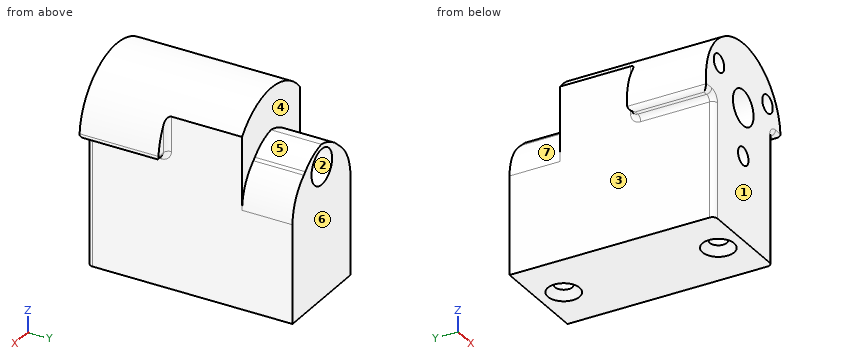
```python
from build123d import *

# Parameters (mm, degrees)
SKETCH2_R                                      = 12.7
BOSS_EXTRUDE6_DEPTH                            = 40.64
SKETCH3_R                                      = 3.5
CUT_EXTRUDE1_DEPTH                             = 40.64
SKETCH4_R                                      = 1.778
CUT_EXTRUDE2_DEPTH                             = 6
BOSS_EXTRUDE8_DEPTH                            = 10
SKETCH8_W                                      = 25.185693912
SKETCH8_H                                      = 10
BOSS_EXTRUDE9_DEPTH                            = 7.284789049
BOSS_EXTRUDE10_DEPTH                           = 30.64
CSK_FOR_M3_FLAT_HEAD_MACHINE_SCREW1_AT_2_COUNT = 2
CSK_FOR_M3_FLAT_HEAD_MACHINE_SCREW1_AT_2_PITCH = 9.039543014
CSK_FOR_M3_FLAT_HEAD_MACHINE_SCREW1_AT_3_COUNT = 2
CSK_FOR_M3_FLAT_HEAD_MACHINE_SCREW1_AT_3_PITCH = 9.039543014
SKETCH16_W                                     = 3.769994858
SKETCH16_H                                     = 22.000968128
CUT_EXTRUDE3_DEPTH                             = 25
SKETCH17_W                                     = 10.276759259
SKETCH17_H                                     = 15.64
CUT_EXTRUDE4_DEPTH                             = 2.743753899
SKETCH18_W                                     = 12.6
SKETCH18_H                                     = 15.64
CUT_EXTRUDE5_DEPTH                             = 2.743753899
SKETCH20_W                                     = 2.743753899
SKETCH20_H                                     = 13.478747573
CUT_EXTRUDE7_DEPTH                             = 25
SKETCH21_W                                     = 5.741451758
SKETCH21_H                                     = 11.696500392
SKETCH21_W_2                                   = 5.938790765
BOSS_EXTRUDE12_DEPTH                           = 15
CUT_EXTRUDE8_START                             = -10
CUT_EXTRUDE8_DEPTH                             = 10
FILLET1_R                                      = 10
FILLET5_R                                      = 10
SKETCH23_W                                     = 2.743753899
SKETCH23_H                                     = 13.478747573
CUT_EXTRUDE9_DEPTH                             = 20
SKETCH24_W                                     = 5.557541457
SKETCH24_H                                     = 9.320824694
SKETCH24_W_2                                   = 5.259690838
BOSS_EXTRUDE13_DEPTH                           = 20
FILLET6_R                                      = 1


with BuildPart() as part:
    # Sketch2 → Boss-Extrude6 (new body)
    with BuildSketch(Plane(origin=(0, -2111.389926236, 0), x_dir=(1, 0, 0), z_dir=(0, 1, 0))):
        with Locations(Location((-53.693967541, 163.840329354, 0), (0, 0, 180))):
            Circle(SKETCH2_R)
    extrude(amount=BOSS_EXTRUDE6_DEPTH)

    # Sketch3 → Cut-Extrude1 (cut)
    with BuildSketch(Plane(origin=(0, -2070.749926236, 0), x_dir=(1, 0, 0), z_dir=(0, 1, 0))):
        with Locations(Location((-53.693967541, 163.840329354, 0), (0, 0, 270))):
            Circle(SKETCH3_R)
    extrude(amount=-CUT_EXTRUDE1_DEPTH, mode=Mode.SUBTRACT)

    # Sketch4 → Cut-Extrude2 (cut)
    with BuildSketch(Plane.XZ.offset(2111.389926236)):
        with Locations(Location((-61.942859512, -159.077829354, 0), (0, 0, 270))):
            Circle(SKETCH4_R)
        with Locations(Location((-53.693967541, -173.365329354, 0), (0, 0, 270))):
            Circle(SKETCH4_R)
        with Locations(Location((-45.44507557, -159.077829354, 0), (0, 0, 270))):
            Circle(SKETCH4_R)
    extrude(amount=-CUT_EXTRUDE2_DEPTH, mode=Mode.SUBTRACT)

    # Sketch7 → Boss-Extrude8 (add)
    with BuildSketch(Plane.XZ.offset(2111.389926236)):
        with BuildLine():
            Line((-40.993967541, -163.840329354), (-40.993967541, -182.634287878))
            Line((-40.993967541, -182.634287878), (-66.179661453, -182.634287878))
            Line((-66.179661453, -182.634287878), (-66.179661453, -166.163570095))
            ThreePointArc((-66.179661453, -166.163570095), (-52.527415502, -176.486639343), (-40.993967541, -163.840329354))
        make_face()
    extrude(amount=-BOSS_EXTRUDE8_DEPTH)

    # Sketch8 → Boss-Extrude9 (add)
    with BuildSketch(Plane(origin=(0, 0, -182.634287878), x_dir=(-1, 0, 0), z_dir=(0, 0, -1))):
        with Locations((53.586814497, -2106.389926236)):
            Rectangle(SKETCH8_W, SKETCH8_H)
    extrude(amount=BOSS_EXTRUDE9_DEPTH)

    # Sketch9 → Boss-Extrude10 (add)
    with BuildSketch(Plane(origin=(0, -2070.749926236, 0), x_dir=(1, 0, 0), z_dir=(0, 1, 0))):
        with BuildLine():
            Line((-66.179661453, 163.840329354), (-66.179661453, 189.919076927))
            Line((-66.179661453, 189.919076927), (-40.993967541, 189.919076927))
            Line((-40.993967541, 189.919076927), (-40.993967541, 163.840329354))
            ThreePointArc((-40.993967541, 163.840329354), (-53.586814497, 176.43317631), (-66.179661453, 163.840329354))
        make_face()
    extrude(amount=-BOSS_EXTRUDE10_DEPTH)

    # Sketch15 → CSK for M3 Flat Head Machine Screw1 (revolve, cut)
    with BuildSketch(Plane(origin=(-53.586814498, -2075.749926236, -189.919076927), x_dir=(0, 1, 0), z_dir=(1, 0, 0))):
        Polygon((0, 0), (0, 10), (1.7, 8.978536948), (1.7, 1.45), (3.15, 0), align=None)
    csk_for_m3_flat_head_machine_screw1 = revolve(axis=Axis((-53.586814498, -2075.749926236, -196.269076927), (0, 0, 1)), mode=Mode.SUBTRACT)

    # CSK for M3 Flat Head Machine Screw1 at 2: CSK for M3 Flat Head Machine Screw1 ×2
    with Locations(*[(-i * CSK_FOR_M3_FLAT_HEAD_MACHINE_SCREW1_AT_2_PITCH, 0, 0) for i in range(1, CSK_FOR_M3_FLAT_HEAD_MACHINE_SCREW1_AT_2_COUNT)]):
        add(csk_for_m3_flat_head_machine_screw1, mode=Mode.SUBTRACT)

    # CSK for M3 Flat Head Machine Screw1 at 3: CSK for M3 Flat Head Machine Screw1 ×2
    with Locations(*[(i * CSK_FOR_M3_FLAT_HEAD_MACHINE_SCREW1_AT_3_PITCH, 0, 0) for i in range(1, CSK_FOR_M3_FLAT_HEAD_MACHINE_SCREW1_AT_3_COUNT)]):
        add(csk_for_m3_flat_head_machine_screw1, mode=Mode.SUBTRACT)

    # Mirror1: CSK for M3 Flat Head Machine Screw1 across plane
    add(csk_for_m3_flat_head_machine_screw1.mirror(Plane.ZX.offset(-2091.069926234)), mode=Mode.SUBTRACT)

    # Mirror1 copy 1 sketch → Mirror1 copy 1 (revolve, cut)
    with BuildSketch(Plane(origin=(-62.626357512, -2106.389926232, -189.919076927), x_dir=(0, -1, 0), z_dir=(1, 0, 0))):
        Polygon((0, 0), (0, -10), (1.7, -8.978536948), (1.7, -1.45), (3.15, 0), align=None)
    revolve(axis=Axis((-62.626357512, -2106.389926232, -196.269076927), (0, 0, -1)), mode=Mode.SUBTRACT)

    # Mirror1 copy 2 sketch → Mirror1 copy 2 (revolve, cut)
    with BuildSketch(Plane(origin=(-44.547271484, -2106.389926232, -189.919076927), x_dir=(0, -1, 0), z_dir=(1, 0, 0))):
        Polygon((0, 0), (0, -10), (1.7, -8.978536948), (1.7, -1.45), (3.15, 0), align=None)
    revolve(axis=Axis((-44.547271484, -2106.389926232, -196.269076927), (0, 0, -1)), mode=Mode.SUBTRACT)

    # Sketch16 → Cut-Extrude3 (cut)
    with BuildSketch(Plane(origin=(0, -2070.749926236, 0), x_dir=(1, 0, 0), z_dir=(0, 1, 0))):
        with Locations((-65.320904983, 165.43984529)):
            Rectangle(SKETCH16_W, SKETCH16_H)
        with Locations((-41.852724011, 165.43984529)):
            Rectangle(SKETCH16_W, SKETCH16_H)
    extrude(amount=-CUT_EXTRUDE3_DEPTH, mode=Mode.SUBTRACT)

    # Sketch17 → Cut-Extrude4 (cut)
    with BuildSketch(Plane.ZY.offset(66.179661453)):
        with Locations((-171.301949724, -2103.569926236)):
            Rectangle(SKETCH17_W, SKETCH17_H)
    extrude(amount=-CUT_EXTRUDE4_DEPTH, mode=Mode.SUBTRACT)

    # Sketch18 → Cut-Extrude5 (cut)
    with BuildSketch(Plane(origin=(-40.993967541, 0, 0), x_dir=(0, 0, -1), z_dir=(1, 0, 0))):
        with Locations((170.140329354, -2103.569926236)):
            Rectangle(SKETCH18_W, SKETCH18_H)
    extrude(amount=-CUT_EXTRUDE5_DEPTH, mode=Mode.SUBTRACT)

    # Sketch20 → Cut-Extrude7 (cut)
    with BuildSketch(Plane(origin=(0, -2070.749926236, 0), x_dir=(1, 0, 0), z_dir=(0, 1, 0))):
        with Locations((-42.365844491, 183.179703141)):
            Rectangle(SKETCH20_W, SKETCH20_H)
        with Locations((-64.807784504, 183.179703141)):
            Rectangle(SKETCH20_W, SKETCH20_H)
    extrude(amount=-CUT_EXTRUDE7_DEPTH, mode=Mode.SUBTRACT)

    # Sketch21 → Boss-Extrude12 (add)
    with BuildSketch(Plane(origin=(0, 0, -189.919076927), x_dir=(-1, 0, 0), z_dir=(0, 0, -1))):
        with Locations((46.608447319, -2076.598176432)):
            Rectangle(SKETCH21_W, SKETCH21_H)
        with Locations((60.466512171, -2076.598176432)):
            Rectangle(SKETCH21_W_2, SKETCH21_H)
    extrude(amount=-BOSS_EXTRUDE12_DEPTH)

    # Sketch22 → Cut-Extrude8 (cut)
    with BuildSketch(Plane(origin=(0, -2070.749926236, 0), x_dir=(1, 0, 0), z_dir=(0, 1, 0)).offset(CUT_EXTRUDE8_START)):
        with BuildLine():
            Line((-49.74995705, 159.255687351), (-53.693967541, 159.255687351))
            Line((-53.693967541, 159.255687351), (-57.324101589, 159.255687351))
            ThreePointArc((-57.324101589, 159.255687351), (-59.615792554, 162.566782678), (-63.435907554, 163.840329354))
            Line((-63.435907554, 163.840329354), (-63.435907554, 159.255687351))
            Line((-63.435907554, 159.255687351), (-63.435907554, 155.692654546))
            ThreePointArc((-63.435907554, 155.692654546), (-53.52421717, 151.141463861), (-43.73772144, 155.95596739))
            Line((-43.73772144, 155.95596739), (-43.73772144, 159.255687351))
            Line((-43.73772144, 159.255687351), (-43.73772144, 163.840329354))
            ThreePointArc((-43.73772144, 163.840329354), (-47.518128803, 162.563400885), (-49.74995705, 159.255687351))
        make_face()
    extrude(amount=CUT_EXTRUDE8_DEPTH, mode=Mode.SUBTRACT)

    # Fillet1
    # the kernel refuses this fillet: 10 mm, written as the material it takes off along each edge
    with BuildSketch(Plane(origin=(-49.74995705, -2080.749926236, -159.255687351), x_dir=(-1, 0, 0), z_dir=(0, 1, 0))) as fillet1_piece_1:
        with BuildLine():
            CenterArc((5.294391522, -10), FILLET1_R, 90, 44.143408643)
            ThreePointArc((-1.670175142, -2.824011483), (-0.645987197, -1.523843369), (0, 0))
            Line((0, 0), (5.294391522, 0))
        make_face()
    extrude(amount=23.235978804, mode=Mode.SUBTRACT)
    with BuildSketch(Plane(origin=(-57.324101589, -2080.749926236, -159.255687351), x_dir=(1, 0, 0), z_dir=(0, 1, 0))) as fillet1_piece_2:
        with BuildLine():
            CenterArc((5.248080135, 10), FILLET1_R, 226.043798631, 43.956201369)
            ThreePointArc((-1.693002689, 2.80129392), (-0.663389254, 1.511313412), (0, 0))
            Line((0, 0), (5.248080135, 0))
        make_face()
    extrude(amount=23.120200338, mode=Mode.SUBTRACT)

    # Fillet5
    fillet5_edges = [part.edges().sort_by_distance(p)[0] for p in [
        (-43.73772144, -2075.749926236, -163.840329354),
        (-63.435907554, -2075.749926236, -163.840329354),
    ]]
    fillet(fillet5_edges, radius=FILLET5_R)

    # Sketch23 → Cut-Extrude9 (cut)
    with BuildSketch(Plane(origin=(0, -2095.749926236, 0), x_dir=(1, 0, 0), z_dir=(0, 1, 0))):
        with Locations((-64.807784504, 183.179703141)):
            Rectangle(SKETCH23_W, SKETCH23_H)
        with Locations((-42.365844491, 183.179703141)):
            Rectangle(SKETCH23_W, SKETCH23_H)
    extrude(amount=-CUT_EXTRUDE9_DEPTH, mode=Mode.SUBTRACT)

    # Sketch24 → Boss-Extrude13 (add)
    with BuildSketch(Plane(origin=(0, 0, -189.919076927), x_dir=(-1, 0, 0), z_dir=(0, 0, -1))):
        with Locations((46.516492169, -2106.729513889)):
            Rectangle(SKETCH24_W, SKETCH24_H)
        with Locations((60.806062135, -2106.729513889)):
            Rectangle(SKETCH24_W_2, SKETCH24_H)
    extrude(amount=-BOSS_EXTRUDE13_DEPTH)

    # Fillet6
    fillet6_edges = [part.edges().sort_by_distance(p)[0] for p in [
        (-63.435907554, -2095.749926236, -160.92811232),
        (-63.435907554, -2111.389926236, -183.17970314),
        (-64.807784503, -2111.389926236, -166.163570095),
        (-63.435907554, -2103.569926236, -166.163570095),
        (-64.807784503, -2095.749926236, -166.163570095),
        (-43.73772144, -2095.749926236, -159.898148372),
        (-42.365844491, -2095.749926236, -163.840329354),
        (-43.73772144, -2103.569926236, -163.840329354),
        (-42.365844491, -2111.389926236, -163.840329354),
        (-43.73772144, -2111.389926236, -183.17970314),
        (-66.179661453, -2103.569926236, -166.163570095),
        (-40.993967541, -2103.569926236, -163.840329354),
    ]]
    fillet(fillet6_edges, radius=FILLET6_R)


solid = part.part
```
The listing builds one solid part. Answer for the finished solid, in the listing's coordinates (mm). Face numbers are marked on the shaded views. A direction names the side the tool comes from. Give positions to 0.01 mm unless a question says otherwise; leave off trailing zeros. Order: outer loops, then holes, each group sorted by start corner. A loop starts at its lowest first (then second) coordinate and runs counter-clockwise, first axis right, second up. Notation, with made-up numbers: (60.5, 4.5) -> (79.5, 4.5) arc R23 cw to (79.5, 20.5) -> close; hole circle Ø3 at (26, 18.5). An arc over 180 degrees is marked (long way). Answer as CSV lines item,"result". Start each with the question number.
Q1. A cutting plane is placed at B-B (y = -2099.5). Determine the outline of the cut face in (x, z).
Q2. A cutting plane is placed at A-A (z = -183). Determine the outline of the cut face in (x, y), then the cut area to 3 significant figures.
Q3. A cutting plane is placed at D-D (x = -61). Determine the outline of the cut face in (y, z), then the cut area to 3 significant figures.
Q4. Which of the six approach directions +Z, -Z, +X, -X, +Y, -Y give full straight-line access (tool end or side, diameter ignored) to the marked faces 4, 5, 6 and 7?
Q5. Determine the mould class of the marked faces 1, 2 and 3 for opening direction X: pulls with the +X half, pulls with the -X half, needs draft (parallel to the pull), parting line crosses it, or undercut.
Q6. A cutting plane is placed at C-C (z = -158.5). Determine the outline of the cut face in (x, y).
Q7. Given pin 1 (1.5 mm diameter, centred on x = -47, z = -159.5, fed in from +Y); pin 2 (0.6 mm diameter, centred on x = -65.5, z = -162.5, fed in from +Y); pin 3 (1.1 mm diameter, centred on x = -53.5, z = -173, fed in from -Y); pin 4 (4 mm diameter, centred on x = -53.69, z = -163.84, fed in from +Y), each flat-ended and moving along its own axis, determine where each tip first touches the part or whether it passes through.
Q8. Find the intervals of material crossed by L1, parallel to Z at x = -53.75, y = -2106; L2, parallel to X at y = -2079, z = -173.5; L3, parallel to Y at x = -50.5, z = -154, in increasing order.
Results found:
1,outline,"(-66.31, -165.28) arc R1 ccw to (-65.32, -166.16) -> (-64.44, -166.16) arc R1 cw to (-63.44, -167.16) -> (-63.44, -189.92) -> (-43.74, -189.92) -> (-43.74, -164.84) arc R1 cw to (-42.74, -163.84) -> (-42.04, -163.84) arc R1 ccw to (-41.04, -162.75) arc R12.7 ccw (long way) to start; hole circle Ø7 at (-53.69, -163.84)"
2,outline,"(-63.44, -2110.39) arc R1 ccw to (-62.44, -2111.39) -> (-44.74, -2111.39) arc R1 ccw to (-43.74, -2110.39) -> (-43.74, -2070.75) -> (-63.44, -2070.75) -> close; hole circle Ø3.4 at (-53.59, -2106.39); hole circle Ø3.4 at (-53.59, -2075.75)"
2,area,"782 mm2"
3,outline,"(-2111.39, -189.92) -> (-2070.75, -189.92) -> (-2070.75, -163.89) -> (-2080.75, -163.89) -> (-2080.75, -153.45) -> (-2111.39, -153.45) -> (-2111.39, -157.57) -> (-2105.39, -157.57) -> (-2105.39, -160.59) -> (-2111.39, -160.59) -> close"
3,area,"1,360 mm2"
4,face 4,"+Z, +Y"
4,face 5,"+Z, +X, +Y"
4,face 6,"+Z, -Z, +X, -X, +Y"
4,face 7,"+Z, -X, +Y"
5,face 1,"needs draft"
5,face 2,"undercut"
5,face 3,"pulls with the -X half"
6,outline,"(-65.22, -2111.39) -> (-63.62, -2111.39) -> (-63.62, -2105.39) -> (-60.26, -2105.39) -> (-60.26, -2111.39) -> (-47.13, -2111.39) -> (-47.13, -2105.39) -> (-43.76, -2105.39) -> (-43.76, -2111.39) -> (-42.17, -2111.39) -> (-42.17, -2095.75) -> (-42.74, -2095.75) arc R1 cw to (-43.74, -2094.75) -> (-43.74, -2080.75) -> (-63.44, -2080.75) -> (-63.44, -2094.75) arc R1 cw to (-64.44, -2095.75) -> (-65.22, -2095.75) -> close"
7,pin 1,"y = -2080.75"
7,pin 2,"y = -2095.75"
7,pin 3,"y = -2105.39"
7,pin 4,"through"
8,L1,"-180.17 to -175.14, -171.59 to -167.34, -160.34 to -151.14"
8,L2,"-63.44 to -43.74"
8,L3,"-2111.39 to -2080.75"
